Design review of the part shown in the three views and the two pictorial views. Dimensions are in mm from the part's minimum x, y and z. Coordinates: 2 decimals unless noted, no trailing zeros. Write each loop counter-clockwise with the first axis right and the second up, starting at its lowest first coordinate (ties: lowest second). Pieces come first, ordered by that corner, then holes.
Q1. Take a section at B-B, the plane z = 0.55. Write out the cut boundary in (x, y), plus the area to 3 significant figures.
Q2. Take a section at A-A, the plane y = 47. Write out the cut boundary in (x, z).
Q3. For pin 1 Ø1 at (y, z) = (26, 2.5) entering from +X; pin 2 Ø12 at (x, y) = (29.5, 39.5) entering from +Z; pin 3 Ø1.6 at (y, z) = (27, 2) entering from -X, all flat-tipped, find the tip position at first contact; note any pin that passes through.
Q4. Take a section at C-C, the plane x = 28. Write out the cut boundary in (y, z).
Q5. The part is to be moulded in two halves that separate along X. For the marked faces 1 and 2, say which applies: released by +X, released by -X, zero draft, split by the parting line, or undercut.
Q6. Take a section at D-D, the plane x = 8. Write out the cut boundary in (y, z).
Q7. For L1, parallel to Y at x = 27.5, z = 2.85; L2, parallel to Y at x = 5, z = 1.5 (1 decimal); L3, parallel to X at y = 29.5, z = 2.7, list the stretches that pass through material, from the lowest coordinate up.
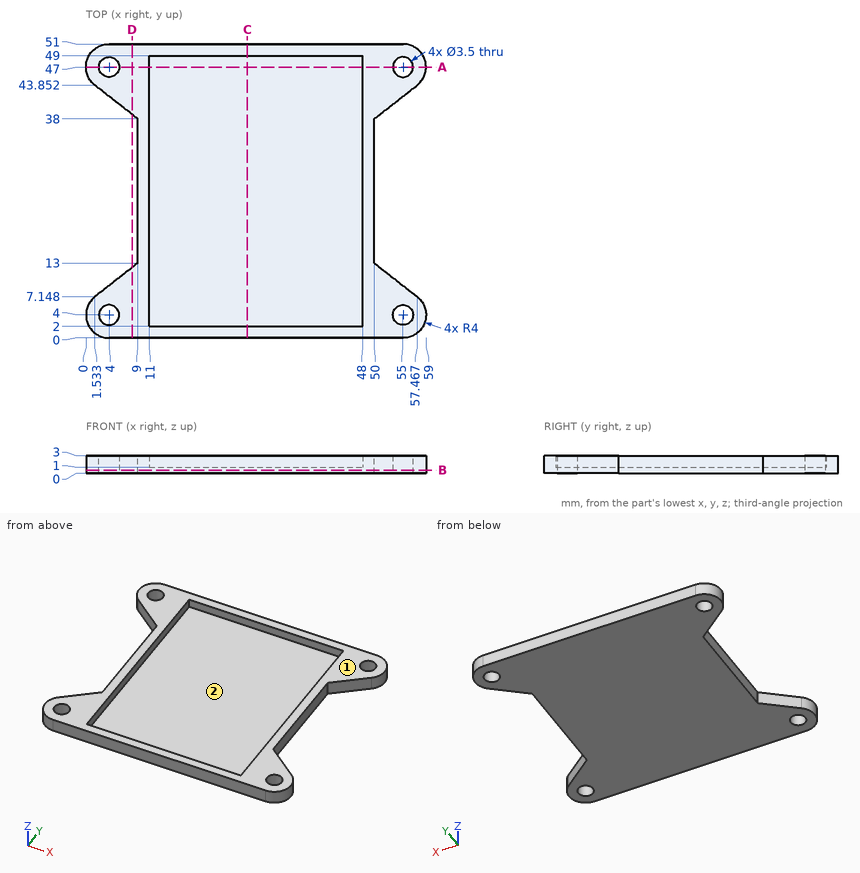
Responses:
1. outline: (1.53, 7.15) arc R4 ccw to (4, 0) - (55, 0) arc R4 ccw to (57.47, 7.15) - (50, 13) - (50, 38) - (57.47, 43.85) arc R4 ccw to (55, 51) - (4, 51) arc R4 ccw to (1.53, 43.85) - (9, 38) - (9, 13) - close; hole circle Ø3.5 at (4, 4); hole circle Ø3.5 at (4, 47); hole circle Ø3.5 at (55, 4); hole circle Ø3.5 at (55, 47)
1. area: 2,380 mm2
2. outline: (0, 0) - (2.25, 0) - (2.25, 3) - (0, 3) - close; (5.75, 0) - (53.25, 0) - (53.25, 3) - (48, 3) - (48, 1) - (11, 1) - (11, 3) - (5.75, 3) - close; (56.75, 0) - (59, 0) - (59, 3) - (56.75, 3) - close
3. pin 1: stops at x = 50
3. pin 2: stops at z = 1
3. pin 3: stops at x = 9
4. outline: (0, 0) - (51, 0) - (51, 3) - (49, 3) - (49, 1) - (2, 1) - (2, 3) - (0, 3) - close
5. face 1: zero draft
5. face 2: undercut
6. outline: (0, 0) - (12.22, 0) - (12.22, 3) - (0, 3) - close; (38.78, 0) - (51, 0) - (51, 3) - (38.78, 3) - close
7. L1: y = 0 to 2, 49 to 51
7. L2: y = 0 to 2.6, 5.4 to 9.9, 41.1 to 45.6, 48.4 to 51
7. L3: x = 9 to 11, 48 to 50
